from build123d import *

# Parameters (mm, degrees)
CROQUIS1_W                 = 5
CROQUIS1_H                 = 13
SALIENTE_EXTRUIR1_DEPTH    = 3
CROQUIS9_R                 = 3.9
SALIENTE_EXTRUIR2_DEPTH    = 30
CROQUIS10_R                = 2
CORTAR_EXTRUIR7_DEPTH      = 45.5
CORTAR_EXTRUIR7_DEPTH_BACK = 45.5


with BuildPart() as part:
    # Croquis1 → Saliente-Extruir1 (new body)
    with BuildSketch(Plane(origin=(0, 0, 0), x_dir=(1, 0, 0), z_dir=(0, 1, 0))):
        Polygon((-45, -26.5), (-30, -26.5), (-30, -44.5), (0, -35.269230769), (30, -44.5), (30, -26.5), (45, -26.5), (45, -7.5), (30, -7.5), (22, 0), (30, 7.5), (45, 7.5), (45, 26.5), (30, 26.5), (30, 44.5), (0, 35.269230769), (-30, 44.5), (-30, 26.5), (-45, 26.5), (-45, 7.5), (-30, 7.5), (-22, 0), (-30, -7.5), (-45, -7.5), align=None)
        Polygon((0, -18.5), (26, -26.5), (26, -39.269230769), (0, -31.269230769), (-26, -39.269230769), (-26, -26.5), align=None, mode=Mode.SUBTRACT)
        Polygon((26, 26.5), (0, 18.5), (-26, 26.5), (-26, 39.269230769), (0, 31.269230769), (26, 39.269230769), align=None, mode=Mode.SUBTRACT)
        with Locations((39.5, -17)):
            Rectangle(CROQUIS1_W, CROQUIS1_H, mode=Mode.SUBTRACT)
        with Locations((39.5, 17)):
            Rectangle(CROQUIS1_W, CROQUIS1_H, mode=Mode.SUBTRACT)
        with Locations((-39.5, 17)):
            Rectangle(CROQUIS1_W, CROQUIS1_H, mode=Mode.SUBTRACT)
        with Locations((-39.5, -17)):
            Rectangle(CROQUIS1_W, CROQUIS1_H, mode=Mode.SUBTRACT)
    extrude(amount=SALIENTE_EXTRUIR1_DEPTH)

    # Croquis9 → Saliente-Extruir2 (add)
    with BuildSketch(Plane(origin=(0, 3, 0), x_dir=(1, 0, 0), z_dir=(0, 1, 0))):
        Circle(CROQUIS9_R)
    extrude(amount=SALIENTE_EXTRUIR2_DEPTH)

    # Croquis10 → Cortar-Extruir7 (cut, two sides)
    with BuildSketch(Plane.XY) as cortar_extruir7_sk:
        with Locations((0, 30)):
            Circle(CROQUIS10_R)
    extrude(amount=CORTAR_EXTRUIR7_DEPTH, mode=Mode.SUBTRACT)
    extrude(cortar_extruir7_sk.sketch, amount=-CORTAR_EXTRUIR7_DEPTH_BACK, mode=Mode.SUBTRACT)


solid = part.part
Could you check a few things on this model? Use its own coordinates, in mm. A direction names the side the tool comes from. Round coordinates to 2 decimals unless told otherwise and drop trailing zeros. Loops run counter-clockwise (first coordinate to the right, second up) from the corner with the lowest first, then second, coordinate; pieces in that order, holes last. Notation, with made-up numbers: (21, -33.5) -> (29, -33.5) arc R22 cw to (29, -0.5) -> close; hole circle Ø7 at (4.5, 27). An arc over 180 degrees is marked (long way). Use CSV: the item, a comma, the result in double quotes.
(1) For faces 4 (the flat face through (42, 1, 17)), 5 (the flat face through (30, 1, 36)), 6 (the cylindrical face through (3.72, 17.79, -1.17)), 7 (the flat face through (25.944, 1.479, -3.698)), which set-ups out of +Z, -Z, +X, -X, +Y, -Y let a thin tool reach every point of the face, with its end or its side?
Return value:
face 4,"+Y, -Y"
face 5,"+Z, +X, +Y, -Y"
face 6,"+Y"
face 7,"+X, +Y, -Y"
(2) Will these pins go through, and if not, where does the flat tip stop? pin 1 Ø1.5 at (x, y) = (-34.5, 1.5) entering from +Z; pin 2 Ø2.5 at (x, y) = (39, 2) entering from -Z; pin 3 Ø3 at (x, y) = (-2.5, 23) entering from -Z; pin 4 Ø1 at (x, z) = (-6.5, -35) entering from -Y.
Return value:
pin 1,"stops at z = 26.5"
pin 2,"stops at z = -26.5"
pin 3,"stops at z = -3.77"
pin 4,"stops at y = 0"
(3) Suppose I cut it at C-C on y = 30. Write out the boundary of the cut face in (x, z).
Return value:
outline,"(-2, -3.35) -> (-2, 3.35) arc R3.9 ccw to start; (2, -3.35) arc R3.9 ccw to (2, 3.35) -> close"
(4) If we mould it in two halves opening along Z, with no side actions, what happens to faces 1 (the flat face through (37, 1, -7.5)), 2 (the cylindrical face through (-1.6, 28.8, 0.1)), 3 (the flat face through (-15.21, 1.48, 39.95))? For each: +Z half, -Z half, draft (parallel to the pull), parting line (faces both ways), or undercut.
Return value:
face 1,"undercut"
face 2,"draft"
face 3,"+Z half"
(5) Suppose I cut it at A-A on x = -31.5. Write out the boundary of the cut face in (y, z), plus the area to 3 significant figures.
Return value:
outline,"(0, -26.5) -> (3, -26.5) -> (3, -7.5) -> (0, -7.5) -> close; (0, 7.5) -> (3, 7.5) -> (3, 26.5) -> (0, 26.5) -> close"
area,"114 mm²"
(6) Suppose I cut it at D-D on x = -5. Write out the boundary of the cut face in (y, z).
Return value:
outline,"(0, -36.81) -> (3, -36.81) -> (3, -32.81) -> (0, -32.81) -> close; (0, -20.04) -> (3, -20.04) -> (3, 20.04) -> (0, 20.04) -> close; (0, 32.81) -> (3, 32.81) -> (3, 36.81) -> (0, 36.81) -> close"
(7) If I drill on probe 1 along Y at (x, z) = (0, 0); probe 2 along X at (y, z) = (30, 0.25); probe 3 along Y at (x, z) = (-19.5, -9.5), over which ranges is the centre line in solid material (lowest first)? Write a range as [from, to].
Return value:
probe 1,"y = [0, 28], [32, 33]"
probe 2,"x = [-3.89, -2], [2, 3.89]"
probe 3,"y = [0, 3]"
(8) Suppose I cut it at B-B on x = 6. Write out the boundary of the cut face in (y, z), plus the area to 3 significant figures.
Return value:
outline,"(0, -37.12) -> (3, -37.12) -> (3, -33.12) -> (0, -33.12) -> close; (0, -20.35) -> (3, -20.35) -> (3, 20.35) -> (0, 20.35) -> close; (0, 33.12) -> (3, 33.12) -> (3, 37.12) -> (0, 37.12) -> close"
area,"146 mm²"
